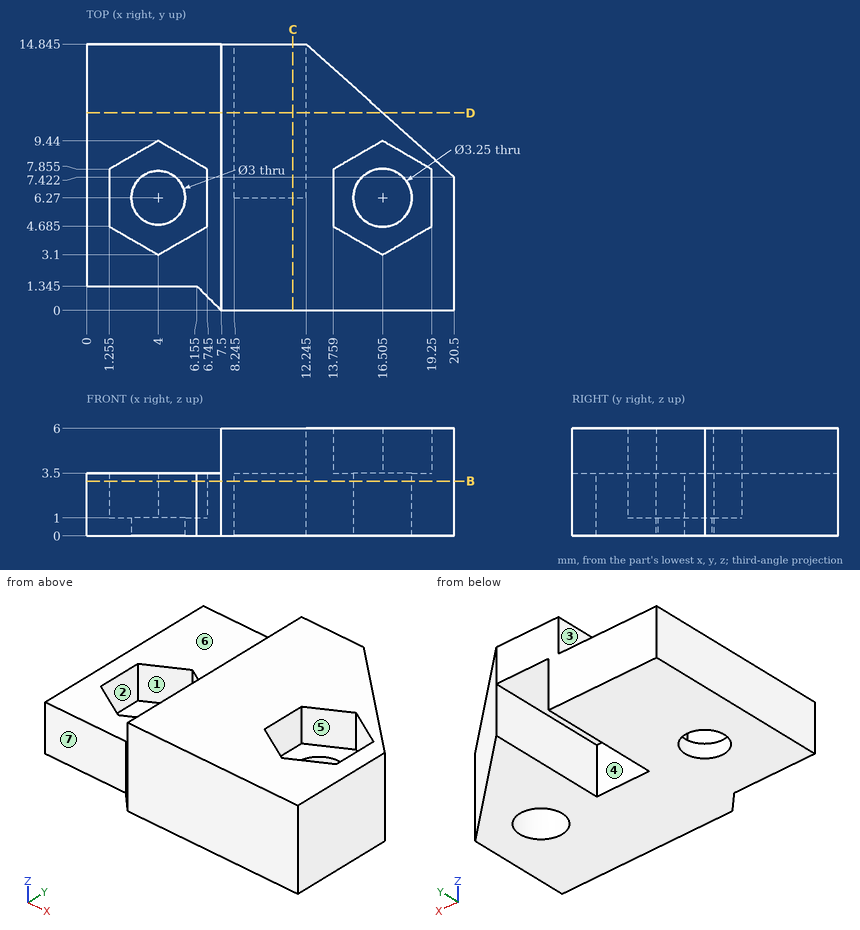
Check sheet for the drawn part. Datum: minimum x, y, z corner. Units: mm. A direction names the side the tool comes from. Round coordinates to 2 decimals unless told otherwise and drop trailing zeros. Order: outer loops, then holes, each group sorted by start corner. A loop starts at its lowest first (then second) coordinate and runs counter-clockwise, first axis right, second up. Notation, with made-up numbers: (40, -3.5) -> (48, -3.5) arc R10 cw to (48, 3.5) -> close; hole circle Ø4 at (79, -30.75). An arc over 180 degrees is marked (long way). Use CSV: the item, a comma, the result in double quotes.
(1) Cross-section at C-C (x = 11.5). Record the boundary of the cut face in (y, z) (1 decimal).
Worked out:
outline,"(0, 0) -> (6.3, 0) -> (6.3, 3.5) -> (14.8, 3.5) -> (14.8, 6) -> (0, 6) -> close"
(2) Cross-section at B-B (z = 3.05). Count the separate pieces of the cut face and the enclosed holes in it, and give its area (3 significant figures).
Worked out:
separate pieces,"1"
enclosed holes,"2"
area,"196 mm²"
(3) Tool access check on the marked faces 5, 6 and 7. Record the directions out of +Z, -Z, +X, -X, +Y, -Y that give a thin tool (end or side, any length) a straight path to the whole face; none if there is none.
Worked out:
face 5,"+Z"
face 6,"+Z, -X, +Y, -Y"
face 7,"+Z, -Z, -X, -Y"
(4) Cross-section at D-D (y = 11). Record the boundary of the cut face in (x, z) (1 decimal).
Worked out:
outline,"(0, 0) -> (8.2, 0) -> (8.2, 3.5) -> (12.2, 3.5) -> (12.2, 0) -> (16.5, 0) -> (16.5, 6) -> (7.5, 6) -> (7.5, 3.5) -> (0, 3.5) -> close"
(5) Depth check by flat-ended pin: pin 1 (1 mm diameter, centred on x = 3.5, z = 1.5, fed in from -Y) (1 decimal); pin 2 (1.2 mm diameter, centred on y = 6.5, z = 5, fed in from -X); pin 3 (3.5 mm diameter, centred on x = 16.5, y = 6.27, fed in from +Z); pin 4 (2.5 mm diameter, centred on x = 4, y = 6.27, fed in from -Z). Enter the tip coordinate at first touch or a pass-through.
Worked out:
pin 1,"y = 1.3"
pin 2,"x = 7.5"
pin 3,"z = 3.5"
pin 4,"through"
(6) Material ranges on line 1 along X through (y, z) = (5.25, 5.65); line 2 along X through (y, z) = (8.75, 1.85) (1 decimal); line 3 along Y through (x, z) = (4, 0.8) (1 decimal), recorded low to high. Write a range as from..to.
Worked out:
line 1,"7.5..13.76, 19.25..20.5"
line 2,"0..2.8, 5.2..8.2, 12.2..19"
line 3,"1.3..4.8, 7.8..14.8"
(7) Draft check along Y on the marked faces 1, 2, 3 and 4. Enter one of: pulls with the +Y half, pulls with the -Y half, needs draft (parallel to the pull), parting line crosses it, or undercut.
Worked out:
face 1,"undercut"
face 2,"undercut"
face 3,"needs draft"
face 4,"pulls with the +Y half"
